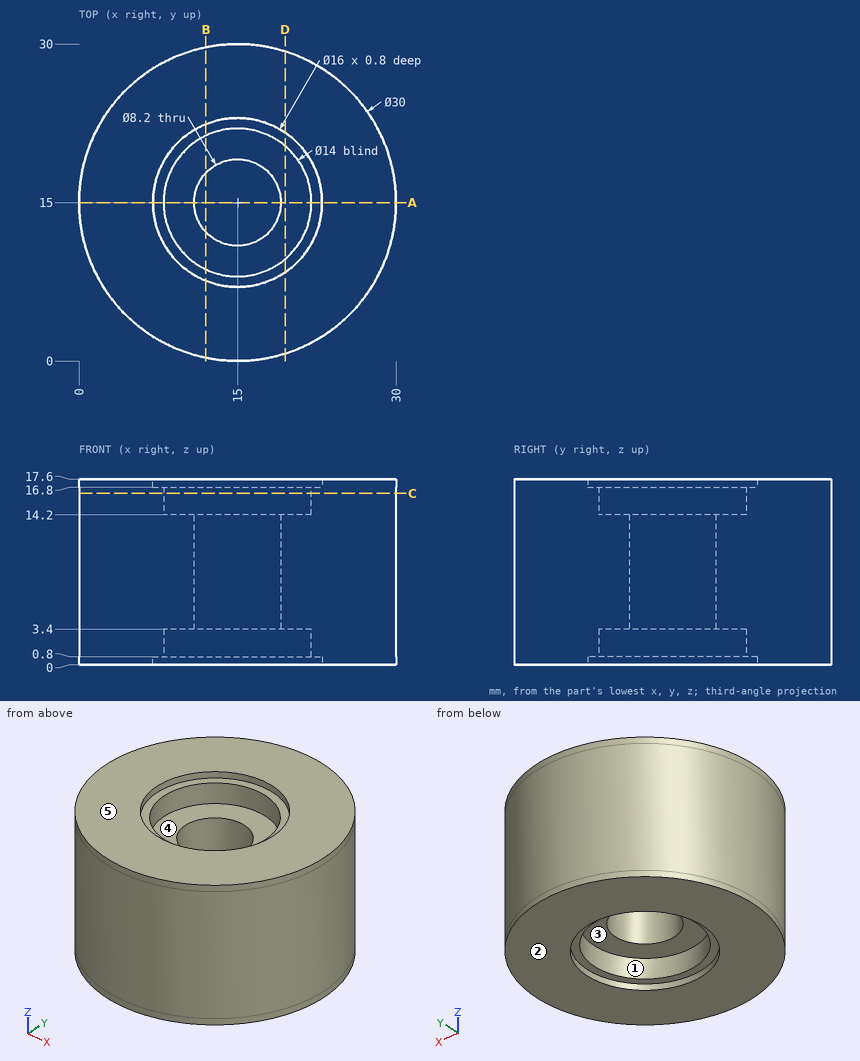
Part print with two shaded views. Sizes in mm from the minimum x, y, z corner. A direction names the side the tool comes from. Round coordinates to 2 decimals unless told otherwise and drop trailing zeros. Write each loop counter-clockwise with the first axis right and the second up, starting at its lowest first coordinate (ties: lowest second). Pieces come first, ordered by that corner, then holes. Notation, with made-up numbers: (35.25, 63) -> (63.25, 63) arc R22 ccw to (63.25, 88) -> close; hole circle Ø7 at (-35.5, 27). An arc over 180 degrees is marked (long way). Use one line per item in the form item = value.
Q1. Band-saw the part on D-D, the plane x = 19.5. Write the cut outline in (y, z), then the cut area to 3 significant figures.
Conclusion:
outline = (0.69, 0) -> (8.39, 0) -> (8.39, 0.8) -> (9.64, 0.8) -> (9.64, 3.4) -> (20.36, 3.4) -> (20.36, 0.8) -> (21.61, 0.8) -> (21.61, 0) -> (29.31, 0) -> (29.31, 17.6) -> (21.61, 17.6) -> (21.61, 16.8) -> (20.36, 16.8) -> (20.36, 14.2) -> (9.64, 14.2) -> (9.64, 16.8) -> (8.39, 16.8) -> (8.39, 17.6) -> (0.69, 17.6) -> close
area = 427 mm²
Q2. Band-saw the part on B-B, the plane x = 12. Write the cut outline in (y, z).
Conclusion:
outline = (0.3, 0) -> (7.58, 0) -> (7.58, 0.8) -> (8.68, 0.8) -> (8.68, 3.4) -> (12.21, 3.4) -> (12.21, 14.2) -> (8.68, 14.2) -> (8.68, 16.8) -> (7.58, 16.8) -> (7.58, 17.6) -> (0.3, 17.6) -> close; (17.79, 3.4) -> (21.32, 3.4) -> (21.32, 0.8) -> (22.42, 0.8) -> (22.42, 0) -> (29.7, 0) -> (29.7, 17.6) -> (22.42, 17.6) -> (22.42, 16.8) -> (21.32, 16.8) -> (21.32, 14.2) -> (17.79, 14.2) -> close
Q3. Drill centre lines: L1, parallel to Y at x = 15, z = 17.25; L2, parallel to Y at x = 15, z = 8; L3, parallel to X at y = 14.5, z = 14.5. Where is each one in solid material? Low to high.
Conclusion:
L1 = 0 to 7, 23 to 30
L2 = 0 to 10.9, 19.1 to 30
L3 = 0.01 to 8.02, 21.98 to 29.99
Q4. Drop flat-ended pins along their axis: P1, Ø4, axis at x = 7.5, z = 4, coming from the +Y side; P2, Ø8.5, axis at x = 15, y = 15, coming from the +Z side; P3, Ø5, axis at x = 17, y = 17, coming from the -Z side. Give the stop position or say it passes through.
Conclusion:
P1 = 28.96
P2 = 14.2
P3 = 3.4
Q5. Two-plate mould, pull along Y, no slides. Class the marked faces 1 and 2: released by +Y, released by -Y, zero draft, split by the parting line, or undercut.
Conclusion:
face_1 = undercut
face_2 = zero draft
Q6. Band-saw the part on C-C, the plane z = 16.25. Write the cut outline in (x, y), then the cut area to 3 significant figures.
Conclusion:
outline = circle Ø30 at (15, 15); hole circle Ø14 at (15, 15)
area = 553 mm²
Q7. Band-saw the part on A-A, the plane y = 15. Write the cut outline in (x, z), then the cut area to 3 significant figures.
Conclusion:
outline = (0, 0) -> (7, 0) -> (7, 0.8) -> (8, 0.8) -> (8, 3.4) -> (10.9, 3.4) -> (10.9, 14.2) -> (8, 14.2) -> (8, 16.8) -> (7, 16.8) -> (7, 17.6) -> (0, 17.6) -> close; (19.1, 3.4) -> (22, 3.4) -> (22, 0.8) -> (23, 0.8) -> (23, 0) -> (30, 0) -> (30, 17.6) -> (23, 17.6) -> (23, 16.8) -> (22, 16.8) -> (22, 14.2) -> (19.1, 14.2) -> close
area = 341 mm²
Q8. Tool access for the marked faces 3, 4 and 5: list every direction of +Z, -Z, +X, -X, +Y, -Y with a clear straight run to the whole face (end or side of a thin tool).
Conclusion:
face_3 = -Z
face_4 = +Z
face_5 = +Z, +X, -X, +Y, -Y
